```python
from build123d import *

# Parameters (mm, degrees)
RECPAT_COUNT = 2
RECPAT_ANGLE = 90


with BuildPart() as part:
    # Fillet1: read off the stored shape, not the designer's step
    # Fillet1 outline → Fillet1 (revolve)
    with BuildSketch(Plane.YX):
        with BuildLine():
            Line((1.5, 2.45), (1.5, 12.35))
            Line((1.5, 12.35), (0, 12.35))
            Line((0, 12.35), (0, 1.65))
            Line((0, 1.65), (3.75, 1.65))
            Line((3.75, 1.65), (3.75, 2.35))
            Line((3.75, 2.35), (1.6, 2.35))
            ThreePointArc((1.6, 2.35), (1.529289322, 2.379289322), (1.5, 2.45))
        make_face()
    revolve(axis=Axis((0, 0, 0), (1, 0, 0)))

    # PanSke → Pan (revolve)
    with BuildSketch(Plane.XY, mode=Mode.PRIVATE) as pan_sk:
        with BuildLine():
            Line((1.65, 3.133289007), (1.65, 0))
            Line((1.65, 0), (0, 0))
            ThreePointArc((0, 0), (0.437709114, 1.770593121), (1.65, 3.133289007))
        make_face()
    revolve(pan_sk.sketch.rotate(Axis((0, 0, 0), (1, 0, 0)), 90), axis=Axis((0, 0, 0), (1, 0, 0)))

    # Sketch3 → Recess section 0
    with BuildSketch(Plane(origin=(0, 0, 0), x_dir=(0, 0, -1), z_dir=(1, 0, 0))):
        with BuildLine():
            Line((-0.37, 1.45), (0.37, 1.45))
            Line((0.37, 1.45), (0.37, -1.45))
            Line((0.37, -1.45), (-0.37, -1.45))
            Line((-0.37, -1.45), (-0.37, 1.45))
        make_face()
    # Sketch4 → Recess section 1
    with BuildSketch(Plane(origin=(1.83, 0, 0), x_dir=(0, 0, -1), z_dir=(1, 0, 0))):
        with BuildLine():
            Line((-0.37, 2.106524682), (0.37, 2.106524682))
            Line((0.37, 2.106524682), (0.37, -2.106524682))
            Line((0.37, -2.106524682), (-0.37, -2.106524682))
            Line((-0.37, -2.106524682), (-0.37, 2.106524682))
        make_face()
    recess = loft(mode=Mode.SUBTRACT)

    # RecPat: Recess ×2 about axis
    recpat_axis = Axis((0, 0, 0), (1, 0, 0))
    for i in range(1, RECPAT_COUNT):
        add(recess.rotate(recpat_axis, i * RECPAT_ANGLE / (RECPAT_COUNT - 1)), mode=Mode.SUBTRACT)

    # RecCorSke → RecessCore (revolve, cut)
    with BuildSketch(Plane.XY, mode=Mode.PRIVATE) as recesscore_sk:
        Polygon((0, 0), (0, 0.877663335), (4.6, 0.556), (4.780655351, 0), align=None)
    revolve(recesscore_sk.sketch.rotate(Axis((-3.175, 0, 0), (1, 0, 0)), 90), axis=Axis((-3.175, 0, 0), (1, 0, 0)), mode=Mode.SUBTRACT)


solid = part.part
```
Geometry: final body of the model. Coordinates: model frame, mm. A direction names the side the tool comes from. Round coordinates to 2 decimals unless told otherwise and drop trailing zeros. Write each loop counter-clockwise with the first axis right and the second up, starting at its lowest first coordinate (ties: lowest second). Pieces come first, ordered by that corner, then holes.
Item 1: Pin query (flat end, axial travel): P1, Ø1, axis at y = -1.5, z = 2.5, coming from the -X side; P2, Ø0.6, axis at y = -1.5, z = 0, coming from the -X side; P3, Ø1, axis at x = 4, y = 0.5, coming from the -Z side; P4, Ø3, axis at y = -1, z = 1, coming from the -X side. Return the tip coordinate at first contact, or that it passes through.
Item 2: Section query C-C (x = 2.75). Return loops of the section in (y, z).
Item 3: Section query B-B (z = -2.25). Return loops of the section in (x, y).
Item 4: Section query A-A (x = 5). Return loops of the section in (y, z), plus the area to 3 significant figures.
Item 5: Set-up query: faces 1 (the face through (7.47, -1.5, 0.07)), 2 (the face through (12.35, 0, 0)). Return all of +Z, -Z, +X, -X, +Y, -Y with unobstructed straight access to the full face (end or side cutting, diameter ignored); none if empty.
Item 6: Mould query, pull axis Z, two halves, no side actions, for faces 3 (the face through (4.77, -0.03, 0)), 4 (the face through (2.882, -0.457, -0.498)), 5 (the face through (2.005, -3.746, 0.165)), 6 (the face through (2.35, 0, -2)). Classes: +Z half, -Z half, draft (parallel to the pull), parting line (faces both ways), or undercut.
Item 7: Material intervals for L1, parallel to X at y = -0.75, z = 0.25; L2, parallel to Y at x = 1.25, z = -0.75; L3, parallel to Y at x = 8.5, z = 1, sorted ascending.
Completed:
1. P1: stops at x = 0.87
1. P2: stops at x = 0.34
1. P3: stops at z = -1.5
1. P4: stops at x = 0.1
2. outline: circle Ø3 at (0, 0); hole circle Ø1.37 at (0, 0)
3. outline: (1.65, -3) - (2.35, -3) - (2.35, 3) - (1.65, 3) - (1.65, 2.18) arc R3.06 ccw to (1.65, -2.18) - close
4. outline: circle Ø3 at (0, 0)
4. area: 7.07 mm2
5. face 1: +X
5. face 2: +Z, -Z, +X, +Y, -Y
6. face 3: undercut
6. face 4: undercut
6. face 5: parting line
6. face 6: draft
7. L1: x = 1.83 to 12.35
7. L2: y = -2.72 to -0.37, 0.37 to 2.72
7. L3: y = -1.12 to 1.12
